from build123d import *

# Parameters (mm, degrees)
BOSS_EXTRUDE1_DEPTH                             = 4.699
CSK_FOR_M3_FLAT_HEAD_MACHINE_SCREW1_D           = 3.4
CSK_FOR_M3_FLAT_HEAD_MACHINE_SCREW1_CSINK_D     = 6.3
CSK_FOR_M3_FLAT_HEAD_MACHINE_SCREW1_CSINK_ANGLE = 90


with BuildPart() as part:
    # Sketch1 → Boss-Extrude1 (new body)
    with BuildSketch(Plane(origin=(0, 0, 0), x_dir=(1, 0, 0), z_dir=(0, 1, 0))):
        with BuildLine():
            Line((-27.186408409, 33.252800217), (24.537514164, 35.252800217))
            ThreePointArc((24.537514164, 35.252800217), (28.016450893, 38.035446755), (26.381150789, 42.179347826))
            ThreePointArc((26.381150789, 42.179347826), (-1.922238221, 49.712850454), (-29.559395906, 40.016304348))
            ThreePointArc((-29.559395906, 40.016304348), (-30.869828758, 35.758501128), (-27.186408409, 33.252800217))
        make_face()
    extrude(amount=BOSS_EXTRUDE1_DEPTH)

    # CSK for M3 Flat Head Machine Screw1 (through all)
    with Locations(Plane(origin=(0, 4.699, 0), x_dir=(1, 0, 0), z_dir=(0, 1, 0))):
        with Locations((-27.331300737, 37), (24.392621835, 39)):
            CounterSinkHole(CSK_FOR_M3_FLAT_HEAD_MACHINE_SCREW1_D / 2, CSK_FOR_M3_FLAT_HEAD_MACHINE_SCREW1_CSINK_D / 2, counter_sink_angle=CSK_FOR_M3_FLAT_HEAD_MACHINE_SCREW1_CSINK_ANGLE)


solid = part.part
Check sheet for the modelled part. Datum: model origin and axes. Units: mm. Give positions to 0.01 mm unless a question says otherwise; leave off trailing zeros. Loops run counter-clockwise (first coordinate to the right, second up) from the corner with the lowest first, then second, coordinate; pieces in that order, holes last. Notation, with made-up numbers: M 2.25,-3.75 L 55.25,-3.75 A23 ccw 55.25,12.25 Z; hole C 55,85.25 d3. An arc over 180 degrees is marked long. Use a Markdown table: item, result. Add a question column.
Q1. Sectioned sample at C-C, the plane z = -44.5. Record the cut outline in (x, y), then the cut area to 3 significant figures.
Q2. Sectioned sample at A-A, the plane y = 2.5. Record the cut outline in (x, z), then the cut area to 3 significant figures.
Q3. Mould release check, pull along Z, two halves, no side actions. Record for faces 1 (the flat face through (-2, 0, -42)), 2 (the cylindrical face through (-25.98, 1.6, -35.97)), 3 (the cylindrical face through (-30.89, 2.32, -35.82)): pulls with the +Z half, pulls with the -Z half, needs draft (parallel to the pull), parting line crosses it, or undercut.
Q4. Scan lines: line 1 along X through (y, z) = (0.6, -37.75); line 2 along X through (y, z) = (1.75, -37); line 3 along X through (y, z) = (3.5, -38.5). Record each from-to range of solid material in increasing order. Write a range as [from, to].
Q5. Go/stop test with flat-tipped pins: pin 1 (4 mm diameter, centred on x = 24.39, z = -39, fed in from -Y); pin 2 (4.5 mm diameter, centred on x = -27.33, z = -37, fed in from +Y); pin 3 (4 mm diameter, centred on x = -19.5, z = -48, fed in from +Y). Record where each tip stops, or that it passes through.
Q6. Sectioned sample at B-B, the plane x = -14.5. Record the cut outline in (y, z).
Verdict:
| question | item | result |
|---|---|---|
| 1 | outline | M -22.24,0 L 22.24,0 L 22.24,4.7 L -22.24,4.7 Z |
| 1 | area | 209 mm^2 |
| 2 | outline | M -29.56,-40.02 A49.75 ccw 26.38,-42.18 A3.75 ccw 24.54,-35.25 L -27.19,-33.25 A3.75 ccw Z; hole C -27.33,-37 d3.4; hole C 24.39,-39 d3.4 |
| 2 | area | 707 mm^2 |
| 3 | face 1 | needs draft |
| 3 | face 2 | undercut |
| 3 | face 3 | parting line crosses it |
| 4 | line 1 | [-31.01, -28.86], [-25.81, 23.24], [25.54, 27.93] |
| 4 | line 2 | [-31.08, -29.03], [-25.63, 27.56] |
| 4 | line 3 | [-30.77, -28.58], [-26.08, 22.51], [26.28, 28.11] |
| 5 | pin 1 | y = 0 |
| 5 | pin 2 | y = 3.8 |
| 5 | pin 3 | through |
| 6 | outline | M 0,-47.59 L 4.7,-47.59 L 4.7,-33.74 L 0,-33.74 Z |
